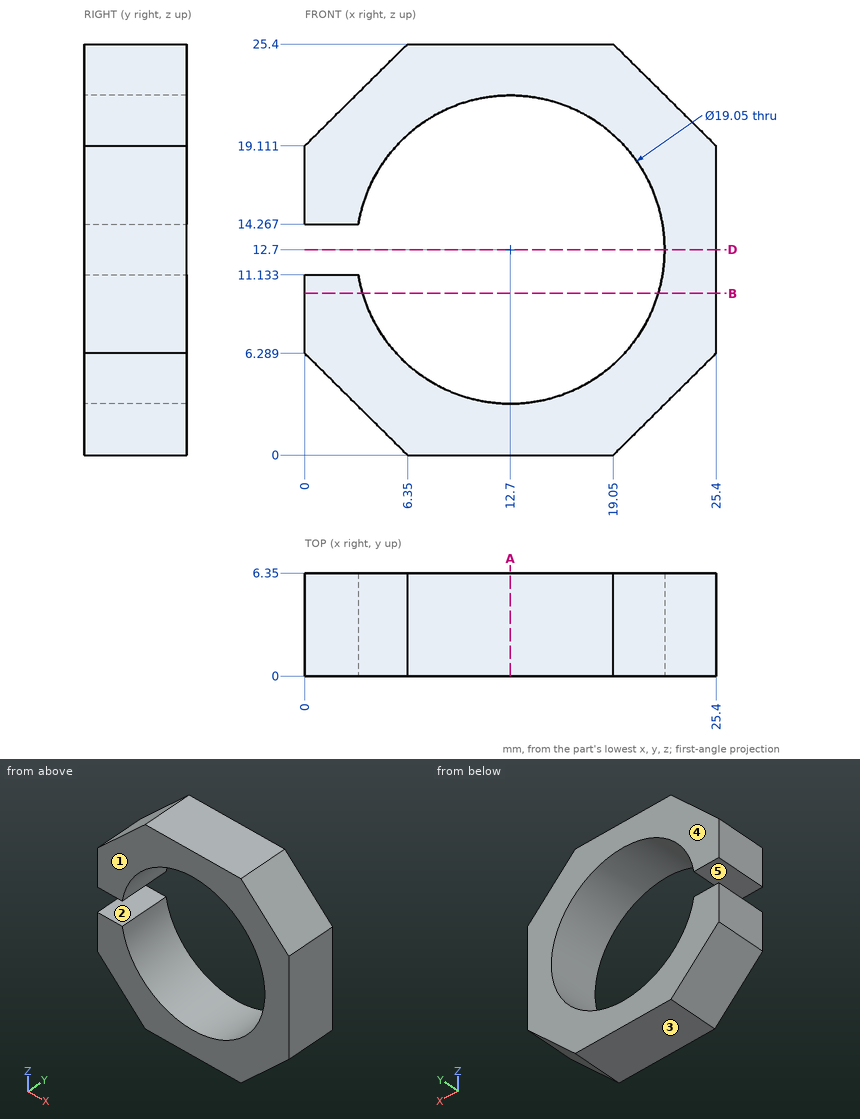
Geometry check sheet. Reference: drawing and pictorial views, mm from the part's lowest x, y, z. A direction names the side the tool comes from. Give positions to 0.01 mm unless a question says otherwise; leave off trailing zeros. Order: outer loops, then holes, each group sorted by start corner. A loop starts at its lowest first (then second) coordinate and runs counter-clockwise, first axis right, second up. Notation, with made-up numbers: (2.5, -39.5) - (6.5, -39.5) arc R21 cw to (6.5, -12.5) - close; hole circle Ø7 at (21, 33). An arc over 180 degrees is marked (long way). Answer as CSV lines item,"result".
1. Section check A-A (x = 12.7). Record the boundary of the cut face in (y, z) (3 decimals).
Result sheet:
outline,"(0, 0) - (6.35, 0) - (6.35, 3.175) - (0, 3.175) - close; (0, 22.225) - (6.35, 22.225) - (6.35, 25.4) - (0, 25.4) - close"
2. Mould release check, pull along Z, two halves, no side actions. Record for the marked faces 1, 2 and 3: released by +Z, released by -Z, zero draft, split by the parting line, or undercut.
Result sheet:
face 1,"zero draft"
face 2,"undercut"
face 3,"released by -Z"
3. Tool access check on the marked faces 4 and 5. Record the directions out of +Z, -Z, +X, -X, +Y, -Y that give a thin tool (end or side, any length) a straight path to the whole face; none if there is none.
Result sheet:
face 4,"+Z, -Z, +X, -X, +Y"
face 5,"-X, +Y, -Y"
4. Scan lines: probe 1 along Z at (x, y) = (13, 4.25); probe 2 along X at (y, z) = (4.75, 6); probe 3 along X at (y, z) = (4.5, 12.7) (3 decimals). Record each from-to range of solid material in increasing order. Write a range as from..to.
Result sheet:
probe 1,"0..3.18, 22.22..25.4"
probe 2,"0.29..5.93, 19.47..25.11"
probe 3,"22.225..25.4"
5. Section check B-B (z = 10). Record the boundary of the cut face in (x, y).
Result sheet:
outline,"(0, 0) - (3.57, 0) - (3.57, 6.35) - (0, 6.35) - close; (21.83, 0) - (25.4, 0) - (25.4, 6.35) - (21.83, 6.35) - close"
6. Section check D-D (z = 12.7). Record the boundary of the cut face in (x, y) (3 decimals).
Result sheet:
outline,"(22.225, 0) - (25.4, 0) - (25.4, 6.35) - (22.225, 6.35) - close"
7. Go/stop test with flat-tipped pins: P1, Ø3.5, axis at x = 2.5, y = 3.5, coming from the -Z side; P2, Ø1.5, axis at y = 2, z = 20.5, coming from the +X side (1 decimal); P3, Ø1.7, axis at x = 2.5, y = 2.5, coming from the +Z side. Record where each tip stops, or that it passes through.
Result sheet:
P1,"z = 2.08"
P2,"x = 24.8"
P3,"z = 22.43"
